```python
from build123d import *

# Parameters (mm, degrees)
EXTRUDE_1_DEPTH     = 5
EXTRUDE_2_DEPTH     = 100
CUT_EXTRUDE_1_DEPTH = 100
CUT_EXTRUDE_2_DEPTH = 100
EXTRUDE_3_DEPTH     = 5
EXTRUDE_4_DEPTH     = 5
SKETCH_9_R          = 2.75
CUT_EXTRUDE_3_DEPTH = 149.07092895


with BuildPart() as part:
    # 草图1 → 凸台-拉伸1 (new body)
    with BuildSketch(Plane(origin=(0, 0, 0), x_dir=(0, 0, -1), z_dir=(1, 0, 0))):
        Polygon((6, 0), (100, 0), (100, -20), (-100, -20), (-100, 0), (-6, 0), (-6, 30), (6, 30), align=None)
    extrude(amount=EXTRUDE_1_DEPTH)

    # 草图2 → 凸台-拉伸2 (add)
    with BuildSketch(Plane(origin=(5, 0, 0), x_dir=(0, 0, -1), z_dir=(1, 0, 0))):
        Polygon((-6, -12), (-6, 30), (6, 30), (6, -12), (100, -12), (100, -20), (-100, -20), (-100, -12), align=None)
    extrude(amount=EXTRUDE_2_DEPTH)

    # 草图3 → 切除-拉伸1 (cut)
    with BuildSketch(Plane(origin=(0, -12, 0), x_dir=(1, 0, 0), z_dir=(0, 1, 0))):
        Polygon((15, 100), (35, 25), (75, 25), (95, 100), align=None)
        Polygon((15, -100), (35, -25), (75, -25), (95, -100), align=None)
    extrude(amount=-CUT_EXTRUDE_1_DEPTH, mode=Mode.SUBTRACT)

    # 草图5 → 切除-拉伸2 (cut)
    with BuildSketch(Plane.XY.offset(6)):
        Polygon((20, 30), (32.5, 0), (77.5, 0), (90, 30), align=None)
    extrude(amount=-CUT_EXTRUDE_2_DEPTH, mode=Mode.SUBTRACT)

    # 草图6 → 凸台-拉伸3 (add)
    with BuildSketch(Plane(origin=(5, 0, 0), x_dir=(0, 0, -1), z_dir=(1, 0, 0))):
        Polygon((-100, 0), (-6, 30), (-6, 0), align=None)
        Polygon((6, 0), (100, 0), (6, 30), align=None)
    extrude(amount=-EXTRUDE_3_DEPTH)

    # 草图7 → 凸台-拉伸4 (add)
    with BuildSketch(Plane(origin=(105, 0, 0), x_dir=(0, 0, -1), z_dir=(1, 0, 0))):
        Polygon((6, 30), (6, -12), (100, -12), (100, 0), align=None)
        Polygon((-100, -12), (-6, -12), (-6, 30), (-100, 0), align=None)
    extrude(amount=-EXTRUDE_4_DEPTH)

    # 草图9 → 切除-拉伸3 (cut, through all)
    with BuildSketch(Plane(origin=(105, 0, 0), x_dir=(0, 0, -1), z_dir=(1, 0, 0))):
        with Locations((30, 8)):
            Circle(SKETCH_9_R)
        with Locations((65, 0)):
            Circle(SKETCH_9_R)
        with Locations((-65, 0)):
            Circle(SKETCH_9_R)
        with Locations((-30, 8)):
            Circle(SKETCH_9_R)
    extrude(amount=-CUT_EXTRUDE_3_DEPTH, mode=Mode.SUBTRACT)


solid = part.part
```
The model under review builds one solid part; all positions refer to its coordinate system, in mm. A direction names the side the tool comes from. Round coordinates to 2 decimals unless told otherwise and drop trailing zeros. Write each loop counter-clockwise with the first axis right and the second up, starting at its lowest first coordinate (ties: lowest second). Pieces come first, ordered by that corner, then holes. Notation, with made-up numbers: (57.5, -7.75) - (74.5, -7.75) arc R21 ccw to (74.5, 4.25) - close; hole circle Ø9 at (-6.5, 18.25). An arc over 180 degrees is marked (long way). Use one line per item in the form item = value.
Q1. For line 1 (X direction, y = 1.5, z = -43); line 2 (Y direction, x = 2.9, z = -30); line 3 (Z direction, x = 12.5, y = -6), list the stretches that pass through material, from the lowest coordinate up. Write a range as [from, to].
Answer key:
line_1 = [0, 5], [100, 105]
line_2 = [-20, 5.25], [10.75, 22.34]
line_3 = [-6, 6]
Q2. Consider section D-D (z = -1). State the section outline as (x, y) points, and give its area (4 significant figures).
Answer key:
outline = (0, -20) - (105, -20) - (105, 30) - (90, 30) - (77.5, 0) - (32.5, 0) - (20, 30) - (0, 30) - close
area = 3,525 mm2
Q3. Consider section C-C (y = -7). State the section outline as (x, z) points.
Answer key:
outline = (0, -100) - (5, -100) - (5, -6) - (100, -6) - (100, -100) - (105, -100) - (105, 100) - (100, 100) - (100, 6) - (5, 6) - (5, 100) - (0, 100) - close
Q4. Insertion check: pin 1 Ø6.5 at (x, y) = (64, -15.5) entering from -Z; pin 2 Ø6.5 at (x, y) = (51, -18) entering from +Z; pin 3 Ø12 at (x, z) = (83.5, 1.5) entering from +Y; pin 4 Ø5 at (y, z) = (0, -65) entering from +X. Each pin has a flat end and moves straight along its axis. Give the tip position at first contact, or say it passes through.
Answer key:
pin_1 = -25
pin_2 = 25
pin_3 = 28.8
pin_4 = through
Q5. Draft analysis for pull direction Y (two halves, no side actions). For faces 1 (the flat face through (10, 30, 0)), 2 (the flat face through (84.86, -15.94, 61.98)), 3 (the cylindrical face through (2.535, 8.121, -27.253)), state which applies: +Y half, -Y half, draft (parallel to the pull), parting line (faces both ways), or undercut.
Answer key:
face_1 = +Y half
face_2 = draft
face_3 = undercut
Q6. Consider section B-B (x = 64). State the section outline as (y, z) points.
Answer key:
outline = (-20, -25) - (-12, -25) - (-12, -6) - (0, -6) - (0, 6) - (-12, 6) - (-12, 25) - (-20, 25) - close
Q7. Consider section A-A (z = -65). State the section outline as (x, y) points.
Answer key:
outline = (0, -20) - (24.33, -20) - (24.33, -12) - (5, -12) - (5, -2.75) - (0, -2.75) - close; (0, 2.75) - (5, 2.75) - (5, 11.17) - (0, 11.17) - close; (85.67, -20) - (105, -20) - (105, -2.75) - (100, -2.75) - (100, -12) - (85.67, -12) - close; (100, 2.75) - (105, 2.75) - (105, 11.17) - (100, 11.17) - close
Q8. Tool access review of faces 4 (the flat face through (52, -12, -21)), 5 (the flat face through (26.162, 15.21, 0.084)), 6 (the flat face through (52, -12, 22)): name each direction out of +Z, -Z, +X, -X, +Y, -Y from which nothing blocks a thin tool from reaching the whole face with its end or side.
Answer key:
face_4 = -Z, +Y
face_5 = +Z, -Z, +Y
face_6 = +Z, +Y
